Autodesk Inventor part; units mm, degrees
ref_plane "YZ Plane" through (0, 0, 0) normal (1, 0, 0) x (0, 1, 0)
ref_plane "XZ Plane" through (0, 0, 0) normal (0, 1, 0) x (-1, 0, 0)
ref_plane "XY Plane" through (0, 0, 0) normal (0, 0, 1) x (1, 0, 0)
sketch "Sketch1" plane through (0, 0, 0) normal (0, 1, 0) x (-1, 0, 0)
  line L0 (0, 0) -> (-68.3, 0) construction
  line L1 (-6.5, 6.5) -> (-61.8, 6.5)
  line L2 (-61.8, -6.5) -> (-6.5, -6.5)
  arc A0 (-6.5, -6.5) -> (-6.5, 6.5) centre (-6.5, 0) ccw
  arc A1 (-61.8, 6.5) -> (-61.8, -6.5) centre (-61.8, 0) ccw
  line L3 (-23.9184, -1.1237) -> (-43.8581, -1.1237) construction
  line L4 (-43.8581, -1.1237) -> (-43.8581, 0.6417) construction
  line L5 (-43.8581, 0.6417) -> (-23.9184, 0.6417) construction
  line L6 (-23.9184, 0.6417) -> (-23.9184, -1.1237) construction
  line L7 (-34.15, -6.5) -> (-34.15, 6.5) construction
  point P0 (-34.15, 0)
  dimension "MinimumRemnant" = 0.9
  dimension "d21" = 68.3
  dimension "d22" = 13
extrude "Plate2" add sketch "Sketch1" against normal blind 0.45
hole "Hole2" at (6.5, 0, 0) at (61.8, 0, 0) direction (0, -1, 0) diameter 4.4958 end through all
equation "\"MinimumRemnant\" = 2 * Thickness"
equation "\"d29\" = Thickness"
equation "\"d23\" = Thickness"
equation "\"BendRadius\" = Thickness"
equation "\"BendReliefWidth\" = Thickness"
equation "\"BendReliefDepth\" = 0.5 * Thickness"
equation "\"CornerReliefSize\" = 4 * Thickness"
equation "\"TransitionRadius\" = BendRadius"
equation "\"JacobiRadiusSize\" = BendRadius"
equation "\"GapSize\" = Thickness"
equation "\"radius\" = 6"
properties part number "Part16.5mm" material "Steel, Carbon"
Model file for the job. Use its own axes, mm. Coordinates: 2 decimals unless noted, no trailing zeros. Order: outer loops, then holes, each group sorted by start corner. A loop starts at its lowest first (then second) coordinate and runs counter-clockwise, first axis right, second up. Notation, with made-up numbers: (-27.75, -16) -> (30.25, -16) arc R30 cw to (30.25, 11) -> close; hole circle Ø3 at (69, 61.5). An arc over 180 degrees is marked (long way). Answer as a JSON object with one key per item and string values. Group by question number.
1) Drill centre lines: L1, parallel to X at y = -0.2, z = 0; L2, parallel to Z at x = 61.8, y = -0.25; L3, parallel to X at y = -0.2, z = -2. Where is each one in solid material? Low to high.
2) Cut at B-B, the plane y = -0.3. Write the cut outline in (x, z), then the cut area to 3 significant figures.
3) Flat gauge pin, fed straight in: pin 1 (2 mm diameter, centred on x = 26.5, z = -4, fed in from +Y). Where does the tip first touch, or does it go through?
4) Cut at C-C, the plane z = 3. Write the cut outline in (x, y).
5) Cut at A-A, the plane z = 0. Write the cut outline in (x, y).
6) Pull direction X, two halves, no side cores. Call faces 1 (the face through (0, -0.2, -0.1)), 2 (the face through (59.57, -0.23, -0.29)), 3 (the face through (8.494, -0.228, 1.037)), 4 (the face through (35, 0, 0)): +X half, -X half, draft (parallel to the pull), parting line (faces both ways), or undercut.
Check values:
{
 "1": {"L1": "x = 0 to 4.25, 8.75 to 59.55, 64.05 to 68.3", "L2": "z = -6.5 to -2.25, 2.25 to 6.5", "L3": "x = 0.32 to 5.47, 7.53 to 60.77, 62.83 to 67.98"},
 "2": {"outline": "(6.5, -6.5) -> (61.8, -6.5) arc R6.5 ccw to (61.8, 6.5) -> (6.5, 6.5) arc R6.5 ccw to start; hole circle Ø4.5 at (6.5, 0); hole circle Ø4.5 at (61.8, 0)", "area": "820 mm²"},
 "3": {"pin 1": "stops at y = 0"},
 "4": {"outline": "(0.73, -0.45) -> (67.57, -0.45) -> (67.57, 0) -> (0.73, 0) -> close"},
 "5": {"outline": "(0, -0.45) -> (4.25, -0.45) -> (4.25, 0) -> (0, 0) -> close; (8.75, -0.45) -> (59.55, -0.45) -> (59.55, 0) -> (8.75, 0) -> close; (64.05, -0.45) -> (68.3, -0.45) -> (68.3, 0) -> (64.05, 0) -> close"},
 "6": {"face 1": "-X half", "face 2": "undercut", "face 3": "undercut", "face 4": "draft"}
}
